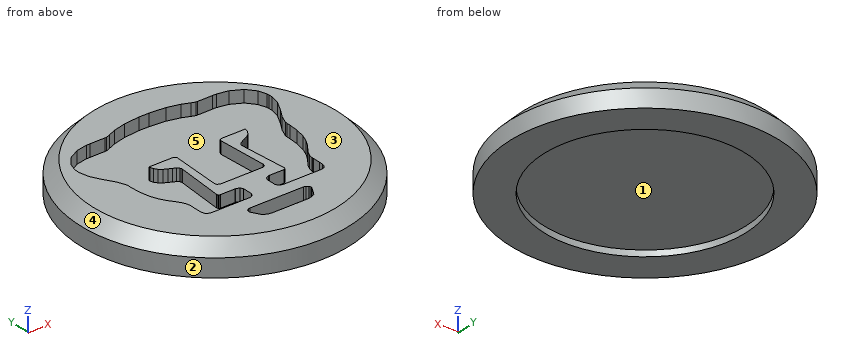
from build123d import *

# Parameters (mm, degrees)
F0_R     = 11
F1_DEPTH = 2.5
F3_DEPTH = 1
F4_SIZE  = 1.016
F5_R     = 8.25
F6_DEPTH = 0.5


with BuildPart() as f1:
    # F0 (on Top) → F1 (new body)
    with BuildSketch(Plane.XY):
        Circle(F0_R)
    extrude(amount=F1_DEPTH)

    # F2 (on face) → F3 (cut)
    with BuildSketch(Plane.XY.offset(2.5)):
        Polygon((-1.708768, -2.738023), (1.709315, -2.738023), (1.765715, -2.730263), (1.942346, -2.632438), (2.000932, -2.453948), (1.998746, -2.405964), (1.780361, 1.612295), (1.778175, 1.651316), (1.84627, 1.782478), (1.99033, 1.835161), (2.038532, 1.835161), (3.923003, 1.835708), (3.919396, 1.748048), (3.844087, 1.485942), (3.665597, 1.225695), (3.421308, 1.032886), (3.146633, 0.884673), (2.876329, 0.758867), (2.645156, 0.63317), (2.48798, 0.48441), (2.43639, 0.337837), (2.440434, 0.290509), (2.766044, -3.632876), (2.767793, -3.656595), (2.719154, -3.757917), (2.626138, -3.811366), (2.595315, -3.811366), (1.421086, -3.81071), (1.347636, -3.810164), (1.078316, -3.917498), (0.956226, -4.145829), (0.956226, -4.222286), (0.956226, -4.871625), (0.956226, -4.947535), (1.086623, -5.177025), (1.330475, -5.277834), (1.411686, -5.277834), (4.284136, -5.276632), (4.351138, -5.276632), (4.553346, -5.267145), (4.772714, -5.201323), (4.920381, -5.023435), (4.974923, -4.76369), (4.974923, -4.677713), (4.974923, -4.460083), (4.977327, -3.881319), (4.974923, -3.808961), (4.970769, -3.706436), (5.029573, -3.396238), (5.202052, -3.035652), (5.452352, -2.678126), (5.739816, -2.27666), (6.026296, -1.783272), (6.271132, -1.150525), (6.434975, -0.33098), (6.485363, 0.461238), (6.478914, 0.72389), (6.511377, 0.956922), (6.786599, 1.630111), (7.273975, 2.429981), (7.711073, 3.274446), (7.8806, 4.055298), (7.868248, 4.312157), (7.85699, 4.532728), (7.643961, 5.185696), (7.080183, 5.888834), (6.195932, 6.359159), (5.306435, 6.529998), (5.010008, 6.529998), (3.774134, 6.530544), (3.665597, 6.530544), (3.340097, 6.648481), (2.725056, 6.907635), (1.690952, 7.167446), (0.422506, 7.284945), (0.000273, 7.284945), (-0.423052, 7.284945), (-1.691608, 7.167446), (-2.725712, 6.908291), (-3.340643, 6.649137), (-3.665707, 6.530544), (-3.773587, 6.530544), (-5.010008, 6.529998), (-5.30709, 6.529998), (-6.196588, 6.359159), (-7.081342, 5.888834), (-7.645273, 5.185696), (-7.857559, 4.532728), (-7.868238, 4.312157), (-7.881288, 4.055298), (-7.711105, 3.274446), (-7.274062, 2.429981), (-6.78661, 1.630111), (-6.51083, 0.956922), (-6.478258, 0.72389), (-6.485363, 0.460692), (-6.435521, -0.33098), (-6.271241, -1.151181), (-6.026405, -1.783819), (-5.739925, -2.277207), (-5.452352, -2.678126), (-5.202707, -3.035652), (-5.03012, -3.396238), (-4.971425, -3.706436), (-4.975032, -3.808961), (-4.977983, -3.881319), (-4.975032, -4.478467), (-4.975032, -4.677713), (-4.975032, -4.76369), (-4.921037, -5.023435), (-4.77337, -5.201323), (-4.554002, -5.267145), (-4.351138, -5.276632), (-4.283589, -5.276632), (-1.411031, -5.277834), (-1.330475, -5.277834), (-1.086623, -5.177025), (-0.956226, -4.947535), (-0.956226, -4.871625), (-0.956226, -4.222286), (-0.956226, -4.145829), (-1.079081, -3.917498), (-1.347636, -3.810164), (-1.420649, -3.81071), (-2.594659, -3.811366), (-2.626138, -3.811366), (-2.719263, -3.757917), (-2.767902, -3.656595), (-2.765498, -3.632876), (-2.439888, 0.290509), (-2.43639, 0.337837), (-2.48798, 0.48441), (-2.644501, 0.63317), (-2.875783, 0.758867), (-3.146742, 0.884673), (-3.421308, 1.032886), (-3.666253, 1.225695), (-3.844743, 1.485942), (-3.919505, 1.748048), (-3.923003, 1.835708), (-2.038422, 1.835161), (-1.990986, 1.835161), (-1.846926, 1.782478), (-1.778175, 1.651316), (-1.779924, 1.612295), (-1.99809, -2.405964), (-2.001151, -2.453948), (-1.942346, -2.632438), (-1.765715, -2.730263), align=None)
        Polygon((-1.357801, -7.715055), (1.358238, -7.715055), (1.462621, -7.715055), (1.776317, -7.664656), (2.092964, -7.50454), (2.138106, -7.449386), (2.511043, -6.796505), (2.530062, -6.761518), (2.551266, -6.635799), (2.500441, -6.488143), (2.361518, -6.379628), (2.194396, -6.337515), (2.139308, -6.337515), (-2.138652, -6.337515), (-2.194943, -6.337515), (-2.362283, -6.379628), (-2.500441, -6.488143), (-2.551375, -6.635799), (-2.530608, -6.761518), (-2.511043, -6.796505), (-2.13745, -7.449386), (-2.092964, -7.50454), (-1.776863, -7.664656), (-1.462621, -7.715055), align=None)
    extrude(amount=-F3_DEPTH, mode=Mode.SUBTRACT)

    # F4
    f4_edges = [f1.edges().sort_by_distance(p)[0] for p in [
        (-11, 0, 2.5),
    ]]
    chamfer(f4_edges, length=F4_SIZE)

    # F5 (on face) → F6 (cut)
    with BuildSketch(Plane(origin=(0, 0, 0), x_dir=(1, 0, 0), z_dir=(0, 0, -1))):
        Circle(F5_R)
    extrude(amount=-F6_DEPTH, mode=Mode.SUBTRACT)


solid = f1.part
Input: part model. Units: mm. Frame: model coordinates. Face numbers are marked on the shaded views. A direction names the side the tool comes from. Round coordinates to 2 decimals unless told otherwise and drop trailing zeros. Loops run counter-clockwise (first coordinate to the right, second up) from the corner with the lowest first, then second, coordinate; pieces in that order, holes last. Notation, with made-up numbers: (24.5, 9.5) -> (55.5, 9.5) arc R18 cw to (55.5, 43.5) -> close; hole circle Ø1 at (9, 43). An arc over 180 degrees is marked (long way). Answer as a JSON object with one key per item and string values. Group by question number.
1) Ray query, L1, parallel to Y at x = 0, z = 0.2; L2, parallel to Y at x = 3.75, z = 2.3; L3, parallel to Z at x = -8, y = 1.5. Return the intervals inside material, ascending.
2) Section query B-B on y = 0. Output: boundary loops of the cut face in (x, z), plus the area to 3 significant figures.
3) Section query A-A on x = 0. Output: boundary loops of the cut face in (y, z).
4) Section query C-C on z = 1.95. State how many separate pieces and enclosed holes the cut face has, plus the area to 3 significant figures.
5) Pin query (flat end, axial travel): pin 1 (5 mm diameter, centred on x = -4.5, y = 1.5, fed in from -Z); pin 2 (1.1 mm diameter, centred on x = 4.5, z = 2, fed in from -Y); pin 3 (1.5 mm diameter, centred on x = -4.5, y = 6.5, fed in from -Z); pin 4 (0.7 mm diameter, centred on x = 0.5, y = -7, fed in from +Z). Return the tip coordinate at first contact, or that it passes through.
6) Section query D-D on z = 0.75. Output: boundary loops of the cut face in (x, y).
7) Reachability of the marked faces 1 and 2 from +Z, -Z, +X, -X, +Y, -Y: full face, straight path, thin tool, end or side. Return the list, or none.
8) Draft query along Y for the marked faces 3, 4 and 5. Return one class per face: +Y half, -Y half, draft (parallel to the pull), parting line (faces both ways), or undercut.
Reply:
{
 "1": {"L1": "y = -11 to -8.25, 8.25 to 11", "L2": "y = -9.47 to -5.28, 1.35 to 1.84, 6.53 to 9.47", "L3": "z = 0.5 to 2.5"},
 "2": {"outline": "(-11, 0) -> (-8.25, 0) -> (-8.25, 0.5) -> (8.25, 0.5) -> (8.25, 0) -> (11, 0) -> (11, 1.48) -> (9.98, 2.5) -> (6.46, 2.5) -> (6.46, 1.5) -> (2.46, 1.5) -> (2.46, 2.5) -> (1.87, 2.5) -> (1.87, 1.5) -> (-1.87, 1.5) -> (-1.87, 2.5) -> (-2.46, 2.5) -> (-2.46, 1.5) -> (-6.46, 1.5) -> (-6.46, 2.5) -> (-9.98, 2.5) -> (-11, 1.48) -> close", "area": "34.0 mm2"},
 "3": {"outline": "(-11, 0) -> (-8.25, 0) -> (-8.25, 0.5) -> (8.25, 0.5) -> (8.25, 0) -> (11, 0) -> (11, 1.48) -> (9.98, 2.5) -> (7.28, 2.5) -> (7.28, 1.5) -> (-2.74, 1.5) -> (-2.74, 2.5) -> (-6.34, 2.5) -> (-6.34, 1.5) -> (-7.72, 1.5) -> (-7.72, 2.5) -> (-9.98, 2.5) -> (-11, 1.48) -> close"},
 "4": {"separate pieces": "1", "enclosed holes": "2", "area": "203 mm2"},
 "5": {"pin 1": "stops at z = 0.5", "pin 2": "stops at y = -10.12", "pin 3": "stops at z = 0", "pin 4": "stops at z = 1.5"},
 "6": {"outline": "circle Ø22 at (0, 0)"},
 "7": {"face 1": "-Z", "face 2": "+Z, -Z"},
 "8": {"face 3": "draft", "face 4": "parting line", "face 5": "undercut"}
}
